```python
from build123d import *

# Parameters (mm, degrees)
SKETCH3_W           = 212
SKETCH3_H           = 130
BOSS_EXTRUDE1_DEPTH = 3
SKETCH4_R           = 2
BOSS_EXTRUDE2_DEPTH = 4
SKETCH5_R           = 1
BOSS_EXTRUDE3_DEPTH = 5
SKETCH6_R           = 2
BOSS_EXTRUDE4_DEPTH = 25
SKETCH7_R           = 1
BOSS_EXTRUDE5_DEPTH = 5
SKETCH8_R           = 16
CUT_EXTRUDE1_DEPTH  = 10


with BuildPart() as part:
    # Sketch3 → Boss-Extrude1 (new body)
    with BuildSketch(Plane(origin=(0, 0, 0), x_dir=(1, 0, 0), z_dir=(0, 1, 0))):
        Rectangle(SKETCH3_W, SKETCH3_H)
    extrude(amount=BOSS_EXTRUDE1_DEPTH)

    # Sketch4 → Boss-Extrude2 (add)
    with BuildSketch(Plane(origin=(0, 3, 0), x_dir=(1, 0, 0), z_dir=(0, 1, 0))):
        with Locations(Location((66, 25, 0), (0, 0, 270))):
            Circle(SKETCH4_R)
        with Locations(Location((66, -22, 0), (0, 0, 270))):
            Circle(SKETCH4_R)
    extrude(amount=BOSS_EXTRUDE2_DEPTH)

    # Sketch5 → Boss-Extrude3 (add)
    with BuildSketch(Plane(origin=(0, 3, 0), x_dir=(1, 0, 0), z_dir=(0, 1, 0))):
        with Locations(Location((-50, 30, 0), (0, 0, 270))):
            Circle(SKETCH5_R)
        with Locations(Location((-1, 30, 0), (0, 0, 270))):
            Circle(SKETCH5_R)
        with Locations(Location((-1, -28, 0), (0, 0, 270))):
            Circle(SKETCH5_R)
        with Locations(Location((-50, -28, 0), (0, 0, 270))):
            Circle(SKETCH5_R)
    extrude(amount=BOSS_EXTRUDE3_DEPTH)

    # Sketch6 → Boss-Extrude4 (add)
    with BuildSketch(Plane(origin=(0, 3, 0), x_dir=(1, 0, 0), z_dir=(0, 1, 0))):
        with Locations(Location((-59, -49, 0), (0, 0, 270))):
            Circle(SKETCH6_R)
        with Locations(Location((-59, 37, 0), (0, 0, 270))):
            Circle(SKETCH6_R)
    extrude(amount=BOSS_EXTRUDE4_DEPTH)

    # Sketch7 → Boss-Extrude5 (add)
    with BuildSketch(Plane(origin=(0, 3, 0), x_dir=(1, 0, 0), z_dir=(0, 1, 0))):
        with Locations(Location((19, 36, 0), (0, 0, 270))):
            Circle(SKETCH7_R)
        with Locations(Location((32, 36, 0), (0, 0, 270))):
            Circle(SKETCH7_R)
        with Locations(Location((32, -30, 0), (0, 0, 270))):
            Circle(SKETCH7_R)
        with Locations(Location((19, -30, 0), (0, 0, 270))):
            Circle(SKETCH7_R)
    extrude(amount=BOSS_EXTRUDE5_DEPTH)

    # Sketch8 → Cut-Extrude1 (cut)
    with BuildSketch(Plane(origin=(0, 3, 0), x_dir=(1, 0, 0), z_dir=(0, 1, 0))):
        with Locations((0, 65)):
            Circle(SKETCH8_R)
    extrude(amount=-CUT_EXTRUDE1_DEPTH, mode=Mode.SUBTRACT)


solid = part.part
```
Work out the finished part from the listing and answer in its coordinate system (mm). A direction names the side the tool comes from. Round coordinates to 2 decimals unless told otherwise and drop trailing zeros. Order: outer loops, then holes, each group sorted by start corner. A loop starts at its lowest first (then second) coordinate and runs counter-clockwise, first axis right, second up.
Q1. A cutting plane is placed at C-C, the plane z = 16. Determine the outline of the cut face in (x, y).
Solution:
outline: (-106, 0) - (106, 0) - (106, 3) - (-106, 3) - close
Q2. A tool of negligible diameter and unlimited length cuts with its end or side. For faces 1 (the cylindrical face through (-57, 15, -37)), 2 (the flat face through (66, 7, -25)), from which of +Z, -Z, +X, -X, +Y, -Y can it reach the whole face along a straight path? Write none if from no direction.
Solution:
face 1: +Y
face 2: +Z, -Z, +X, -X, +Y
Q3. A cutting plane is placed at A-A, the plane y = 17.75. Determine the outline of the cut face in (x, z), then the cut area to 3 significant figures.
Solution:
outline: circle Ø4 at (-59, -37); circle Ø4 at (-59, 49)
area: 25.1 mm2
Q4. The mould has two halves that part along Z. Classify faces 3 (the cylindrical face through (-57, 15, 49)), 4 (the cylindrical face through (68, 5, 22)), 5 (the flat face through (-59, 28, 49)), 6 (the cylindrical face through (0, 2, -49)): pulls with the +Z half, pulls with the -Z half, needs draft (parallel to the pull), parting line crosses it, or undercut.
Solution:
face 3: undercut
face 4: undercut
face 5: needs draft
face 6: pulls with the -Z half
Q5. A cutting plane is placed at B-B, the plane x = -73. Determine the outline of the cut face in (y, z).
Solution:
outline: (0, -65) - (3, -65) - (3, 65) - (0, 65) - close
Q6. Find the intervals of material crossed by line 1 along Y through (x, z) = (79, 28.5); line 2 along X through (y, z) = (10.25, -38), in increasing order.
Solution:
line 1: y = 0 to 3
line 2: x = -60.73 to -57.27
Q7. Given pin 1 Ø1.5 at (x, z) = (-25.5, -18.5) entering from +Y; pin 2 Ø1 at (x, z) = (19, 30) entering from +Y; pin 3 Ø4.5 at (x, z) = (66, 22) entering from +Y, each flat-ended and moving along its own axis, determine where each tip first touches the part or whether it passes through.
Solution:
pin 1: stops at y = 3
pin 2: stops at y = 8
pin 3: stops at y = 7
